Read the model definition and answer for the solid it produces. Units are mm, in the model's axes. A direction names the side the tool comes from. Give positions to 0.01 mm unless a question says otherwise; leave off trailing zeros. Loops run counter-clockwise (first coordinate to the right, second up) from the corner with the lowest first, then second, coordinate; pieces in that order, holes last. Notation, with made-up numbers: (-40, 72.5) -> (-34, 72.5) arc R28 ccw to (-34, 95.5) -> close; hole circle Ø1 at (55.5, 31.25). An arc over 180 degrees is marked (long way). Answer as CSV lines item,"result". Start each with the question number.
```python
from build123d import *

# Parameters (mm, degrees)
ESTRUSIONE_ESTRUSIONE2_DEPTH  = 74
RACCORDO3_R                   = 15
RACCORDO4_R                   = 2
SCHIZZO10_R                   = 1.7
TAGLIO_ESTRUSIONE1_DEPTH      = 10
SCHIZZO13_R                   = 1.7
TAGLIO_ESTRUSIONE3_DEPTH      = 11.491186204
TAGLIO_ESTRUSIONE3_DEPTH_BACK = 86.53385939


with BuildPart() as part:
    # Schizzo2 → Estrusione-Estrusione2 (new body)
    with BuildSketch(Plane.XY):
        Polygon((-60, 40.884860172), (20.66, 40.884860172), (20.66, 38.384860172), (-58.319751134, 38.384860172), (-69.015504429, 12.162557341), (-71.330346702, 13.1067529), align=None)
    extrude(amount=ESTRUSIONE_ESTRUSIONE2_DEPTH)

    # Raccordo3
    raccordo3_edges = [part.edges().sort_by_distance(p)[0] for p in [
        (-60, 40.884860172, 37),
        (-58.319751134, 38.384860172, 37),
    ]]
    fillet(raccordo3_edges, radius=RACCORDO3_R)

    # Raccordo4
    raccordo4_edges = [part.edges().sort_by_distance(p)[0] for p in [
        (-70.172925565, 12.63465512, 74),
        (-70.172925565, 12.63465512, 0),
    ]]
    fillet(raccordo4_edges, radius=RACCORDO4_R)

    # Schizzo10 → Taglio-Estrusione1 (cut)
    with BuildSketch(Plane(origin=(0, 40.884860172, 0), x_dir=(1, 0, 0), z_dir=(0, 1, 0))):
        with Locations((5.081493197, -67)):
            Circle(SCHIZZO10_R)
        with Locations((5.081493197, -7)):
            Circle(SCHIZZO10_R)
        with Locations((-44.918506803, -67)):
            Circle(SCHIZZO10_R)
        with Locations((-44.918506803, -7)):
            Circle(SCHIZZO10_R)
    extrude(amount=-TAGLIO_ESTRUSIONE1_DEPTH, mode=Mode.SUBTRACT)

    # Schizzo13 → Taglio-Estrusione3 (cut, two sides)
    with BuildSketch(Plane(origin=(-65.73923894, 26.814223222, 0), x_dir=(0, 0, 1), z_dir=(-0.925936909, 0.377678223, 0))) as taglio_estrusione3_sk:
        with Locations((4, -6.803892348)):
            Circle(SCHIZZO13_R)
        with Locations((70, -6.803892348)):
            Circle(SCHIZZO13_R)
        with Locations((35, -6.803892348)):
            Circle(SCHIZZO13_R)
    extrude(amount=TAGLIO_ESTRUSIONE3_DEPTH, mode=Mode.SUBTRACT)
    extrude(taglio_estrusione3_sk.sketch, amount=-TAGLIO_ESTRUSIONE3_DEPTH_BACK, mode=Mode.SUBTRACT)


solid = part.part
```
(1) Find the intervals of material crossed by line 1 along X through (y, z) = (39.6, 67); line 2 along X through (y, z) = (38.9, 7); line 3 along Y through (x, z) = (-2, 57.5), in increasing order. Write a range as from..to.
(2) Find section C-C on x = -8. Write down the section's boundary in (y, z), then the cut area to 3 significant figures.
(3) Each of these flat-tipped pins is pushed along its axis until it touches: P1, Ø12, axis at y = 34, z = 42.5, coming from the -X side; P2, Ø8, axis at y = 36, z = 15.5, coming from the -X side; P3, Ø2, axis at y = 19, z = 29, coming from the -X side; P4, Ø4, axis at x = 5.08, z = 67, coming from the +Y side. Where does it stop, or does it pass through?
(4) Find section B-B on z = 23. Write down the section's boundary in (x, y).
(5) Find section D-D on y = 23.5. Write down the section's boundary in (x, z), then the cut area to 3 significant figures.
(6) A tool of negligible diameter and unlimited length cuts with its end or side. For faces 1 (the face through (-69.96, 13.2, 0.57)), 2 (the face through (-13, 38.385, 36)), from which of +Z, -Z, +X, -X, +Y, -Y can it reach the whole face along a straight path? Write none if from no direction.
(7) Find section A-A on z = 67. Write down the section's boundary in (x, y).
(8) The mould has two halves that part along Y. Classify faces 3 (the face through (-28, 39, 74)), 4 (the face through (-67.1, 20.1, 68.3)), 5 (the face through (-56.502, 35.903, 37.518)): pulls with the +Y half, pulls with the -Y half, needs draft (parallel to the pull), parting line crosses it, or undercut.
Answer block:
1,line 1,"x = -55.99..-46.62, -43.22..3.38, 6.78..20.66"
1,line 2,"x = -57.38..-46.62, -43.22..3.38, 6.78..20.66"
1,line 3,"y = 38.38..40.88"
2,outline,"(38.38, 0) -> (40.88, 0) -> (40.88, 74) -> (38.38, 74) -> close"
2,area,"185 mm2"
3,P1,"stops at x = -65.26"
3,P2,"stops at x = -63.62"
3,P3,"stops at x = -69.33"
3,P4,"stops at y = 40.88"
4,outline,"(-71.33, 13.11) -> (-69.02, 12.16) -> (-62.13, 29.05) arc R15 cw to (-48.24, 38.38) -> (20.66, 38.38) -> (20.66, 40.88) -> (-49.92, 40.88) arc R15 ccw to (-63.81, 31.55) -> close"
5,outline,"(-67.09, 0) -> (-64.39, 0) -> (-64.39, 74) -> (-67.09, 74) -> close"
5,area,"200 mm2"
6,face 1,"-Z, -X, -Y"
6,face 2,"+Z, -Z, +X, -Y"
7,outline,"(-71.33, 13.11) -> (-69.02, 12.16) -> (-62.13, 29.05) arc R15 cw to (-48.24, 38.38) -> (-46.62, 38.38) -> (-46.62, 40.88) -> (-49.92, 40.88) arc R15 ccw to (-63.81, 31.55) -> close; (-43.22, 38.38) -> (3.38, 38.38) -> (3.38, 40.88) -> (-43.22, 40.88) -> close; (6.78, 38.38) -> (20.66, 38.38) -> (20.66, 40.88) -> (6.78, 40.88) -> close"
8,face 3,"needs draft"
8,face 4,"undercut"
8,face 5,"pulls with the -Y half"
